from build123d import *

# Parameters (mm, degrees)
F0_R     = 4
F1_DEPTH = 147
F3_DEPTH = 20
F4_DEPTH = 30


with BuildPart() as f1:
    # F0 (on Front) → F1 (new body, symmetric)
    with BuildSketch(Plane.XZ):
        Circle(F0_R)
    extrude(amount=F1_DEPTH, both=True)

    # F2 (on face) → F3 (cut)
    with BuildSketch(Plane.XZ.offset(147)):
        with BuildLine():
            Line((-3.4641016151, 2), (3.4641016151, 2))
            ThreePointArc((3.4641016151, 2), (0, 4), (-3.4641016151, 2))
        make_face()
    extrude(amount=-F3_DEPTH, mode=Mode.SUBTRACT)

    # F4 (cut): a face of the model
    f4_faces = [f1.faces().sort_by_distance(p)[0] for p in [
        (0, 147, 0),
    ]]
    extrude(f4_faces, amount=-F4_DEPTH, mode=Mode.SUBTRACT)


solid = f1.part
Verification items for the finished model (mm, model axes). A direction names the side the tool comes from. Coordinates: 2 decimals unless noted, no trailing zeros. Order: outer loops, then holes, each group sorted by start corner. A loop starts at its lowest first (then second) coordinate and runs counter-clockwise, first axis right, second up. Notation, with made-up numbers: (49, 29) -> (68, 29) arc R20 cw to (68, 68) -> close; hole circle Ø9 at (-26.75, 20). An arc over 180 degrees is marked (long way). Put each result on its own line as item: value. Start each with the question number.
1. Material ranges on L1, parallel to X at y = 12, z = 0.5; L2, parallel to Z at x = 2, y = 9.5; L3, parallel to Y at x = -0.75, z = 3, recorded low to high. Write a range as [from, to].
2. Access from +Z, -Z, +X, -X, +Y, -Y to the whole of each face (thin tool, end or side, straight path). Record for faces 1 (the flat face through (0, -137, 2)), 2 (the flat face through (0, 117, 0)).
3. Cross-section at A-A, the plane x = 0. Record the boundary of the cut face in (y, z), then the cut area to 3 significant figures.
4. Go/stop test with flat-tipped pins: pin 1 Ø2 at (y, z) = (-115.5, -2.5) entering from +X; pin 2 Ø0.6 at (x, z) = (1.5, 3.5) entering from -Y; pin 3 Ø1.5 at (x, y) = (3, -24.5) entering from +Z. Record where each tip stops, or that it passes through.
5. Cross-section at B-B, the plane y = 85.5. Record the boundary of the cut face in (x, z), then the cut area to 3 significant figures.
Computed:
1. L1: [-3.97, 3.97]
1. L2: [-3.46, 3.46]
1. L3: [-127, 117]
2. face 1: +Z, +X, -X, -Y
2. face 2: +Z, -Z, +X, -X, +Y
3. outline: (-147, -4) -> (117, -4) -> (117, 4) -> (-127, 4) -> (-127, 2) -> (-147, 2) -> close
3. area: 2,070 mm2
4. pin 1: x = 3.71
4. pin 2: y = -127
4. pin 3: z = 3.31
5. outline: circle Ø8 at (0, 0)
5. area: 50.3 mm2
